For this review, use the dimensioned drawing (mm, ordinates from the lowest corner) and the shaded views. A direction names the side the tool comes from. Give positions to 0.01 mm unless a question says otherwise; leave off trailing zeros. Order: outer loops, then holes, each group sorted by start corner. A loop starts at its lowest first (then second) coordinate and runs counter-clockwise, first axis right, second up.
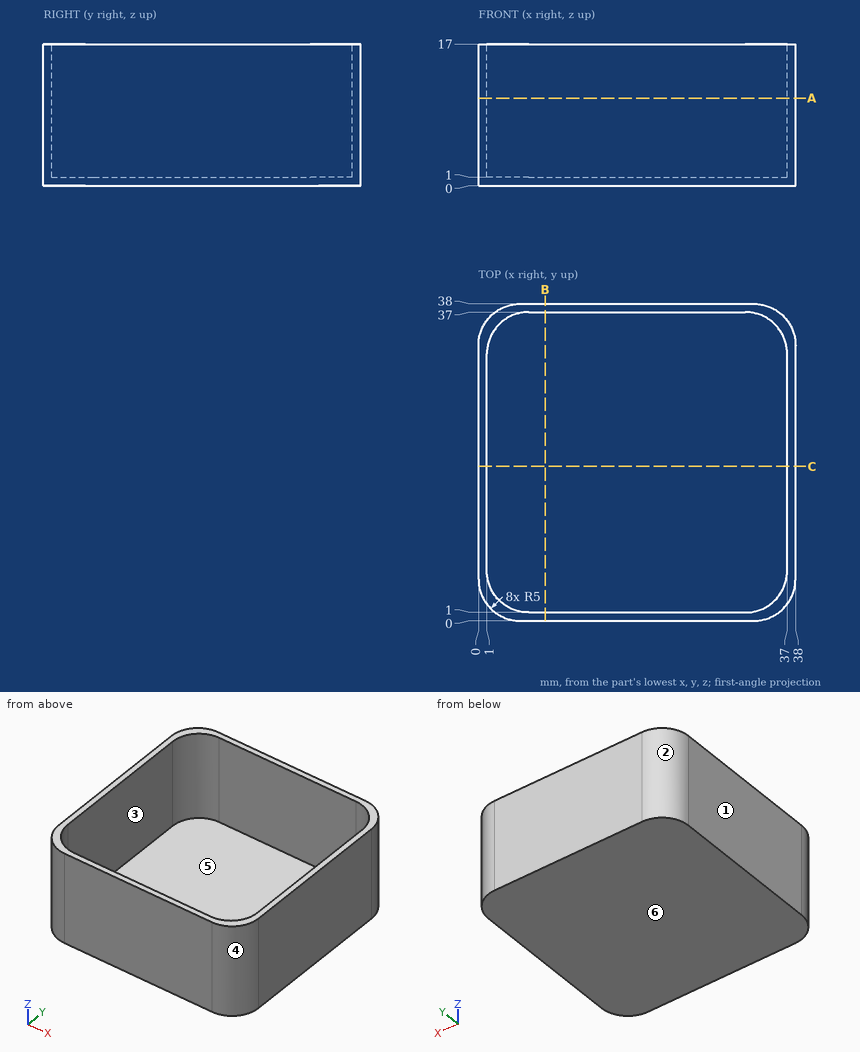
1. Take a section at B-B (x = 8). State the section outline as (y, z) points.
Recorded:
outline: (0, 0) - (38, 0) - (38, 17) - (37, 17) - (37, 1) - (1, 1) - (1, 17) - (0, 17) - close
2. Machinability: for the marked faces 5 and 6, which of the approach directions +Z, -Z, +X, -X, +Y, -Y give a long, thin tool a straight path to every point of the face, cutting with its end or side? Answer none if there is none.
Recorded:
face 5: +Z
face 6: -Z, +X, -X, +Y, -Y
3. For pin 1 (1 mm diameter, centred on x = 17.5, z = 12, fed in from -Y); pin 2 (18 mm diameter, centred on x = 21.5, y = 27.5, fed in from +Z), all flat-tipped, find the tip position at first contact; note any pin that passes through.
Recorded:
pin 1: stops at y = 0
pin 2: stops at z = 1
4. For line 1 along X through (y, z) = (17, 13.5); line 2 along Z through (x, y) = (11.5, 32), list the stretches that pass through material, from the lowest coordinate up.
Recorded:
line 1: x = 0 to 1, 37 to 38
line 2: z = 0 to 1
5. Take a section at A-A (z = 10.5). State the section outline as (x, y) points.
Recorded:
outline: (0, 5) arc R5 ccw to (5, 0) - (33, 0) arc R5 ccw to (38, 5) - (38, 33) arc R5 ccw to (33, 38) - (5, 38) arc R5 ccw to (0, 33) - close; hole (1, 6) arc R5 ccw to (6, 1) - (32, 1) arc R5 ccw to (37, 6) - (37, 32) arc R5 ccw to (32, 37) - (6, 37) arc R5 ccw to (1, 32) - close
6. Draft analysis for pull direction Y (two halves, no side actions). For the marked faces 1, 2, 3 and 4, state which applies: pulls with the +Y half, pulls with the -Y half, needs draft (parallel to the pull), parting line crosses it, or undercut.
Recorded:
face 1: needs draft
face 2: pulls with the +Y half
face 3: undercut
face 4: pulls with the -Y half
